```python
from build123d import *

# Parameters (mm, degrees)
ESBO_O1_W                = 4
ESBO_O1_H                = 3.5
ESBO_O2_R                = 2
RESSALTO_EXTRUS_O1_DEPTH = 16
CORTE_EXTRUS_O1_DEPTH    = 2
CHANFRO1_SIZE            = 0.39
FILETE1_R                = 0.2


with BuildPart() as part:
    # Esboço1 → Revolução1 (revolve)
    with BuildSketch(Plane(origin=(0, 0, 0), x_dir=(-1, 0, 0), z_dir=(0, 0, -1))):
        with Locations((-2, 1.75)):
            Rectangle(ESBO_O1_W, ESBO_O1_H)
    revolve(axis=Axis((4, 0, 0), (-1, 0, 0)))

    # Esboço2 → Ressalto-extrusão1 (add)
    with BuildSketch(Plane(origin=(4, 0, 0), x_dir=(0, 0, -1), z_dir=(1, 0, 0))):
        Circle(ESBO_O2_R)
    extrude(amount=RESSALTO_EXTRUS_O1_DEPTH)

    # Esboço3 → Corte-extrusão1 (cut)
    with BuildSketch(Plane.ZY):
        Polygon((0, -1.773042677), (1.5355, -0.886521338), (1.5355, 0.886521338), (0, 1.773042677), (-1.5355, 0.886521338), (-1.5355, -0.886521338), align=None)
    extrude(amount=-CORTE_EXTRUS_O1_DEPTH, mode=Mode.SUBTRACT)

    # Esboço4 → Corte-Revolução1 (revolve, cut)
    with BuildSketch(Plane.XY):
        Polygon((2, 1.5355), (2, 0), (2.886521338, 0), align=None)
    revolve(axis=Axis((2, 0, 0), (1, 0, 0)), mode=Mode.SUBTRACT)

    # Chanfro1
    chanfro1_edges = [part.edges().sort_by_distance(p)[0] for p in [
        (20, 0, 2),
    ]]
    chamfer(chanfro1_edges, length=CHANFRO1_SIZE)

    # Filete1
    filete1_edges = [part.edges().sort_by_distance(p)[0] for p in [
        (0, -3.5, 0),
        (4, 0, 2),
    ]]
    fillet(filete1_edges, radius=FILETE1_R)


solid = part.part
```
Part model, mm, in its own coordinate system. A direction names the side the tool comes from. Round coordinates to 2 decimals unless told otherwise and drop trailing zeros. Write each loop counter-clockwise with the first axis right and the second up, starting at its lowest first coordinate (ties: lowest second). Pieces come first, ordered by that corner, then holes.
Item 1: Two-plate mould, pull along Y, no slides. Class faces 1 (the flat face through (0.986, 1.336, -0.757)), 2 (the cylindrical face through (2.073, 3.233, 1.341)), 3 (the flat face through (20, 0, 0)): +Y half, -Y half, draft (parallel to the pull), parting line (faces both ways), or undercut.
Results:
face 1: undercut
face 2: parting line
face 3: draft
Item 2: Drop flat-ended pins along their axis: pin 1 Ø1 at (y, z) = (1, -2) entering from +X; pin 2 Ø0.9 at (x, y) = (0.5, 0.5) entering from +Z; pin 3 Ø3 at (x, z) = (17.5, 0) entering from +Y; pin 4 Ø1 at (x, y) = (14.5, 1.5) entering from +Z. Give the stop position or say it passes through.
Results:
pin 1: stops at x = 19.87
pin 2: stops at z = 3.5
pin 3: stops at y = 2
pin 4: stops at z = 1.73
Item 3: Cut at A-A, the plane x = 18.25. Give the cut face in (y, z).
Results:
outline: circle Ø4 at (0, 0)
Item 4: Which spindle directions (+Z, -Z, +X, -X, +Y, -Y) get a long thin tool onto all of the face, cutting with end or side? Do faces 4 (the flat face through (4, 2, 2)), 5 (the flat face through (1, 0, -1.536)), 6 (the flat face through (0, 2, 1)). Say none if no direction does.
Results:
face 4: +X
face 5: -X
face 6: +Z, -Z, -X, +Y, -Y
Item 5: Probe L1, parallel to Y at x = 12.75, z = 0; L2, parallel to X at y = -2.5, z = -2; L3, parallel to Y at x = 1.75, z = 1. List the from-to ranges inside material, lowest first.
Results:
L1: y = -2 to 2
L2: x = 0 to 4
L3: y = -3.35 to -1.2, 1.2 to 3.35
